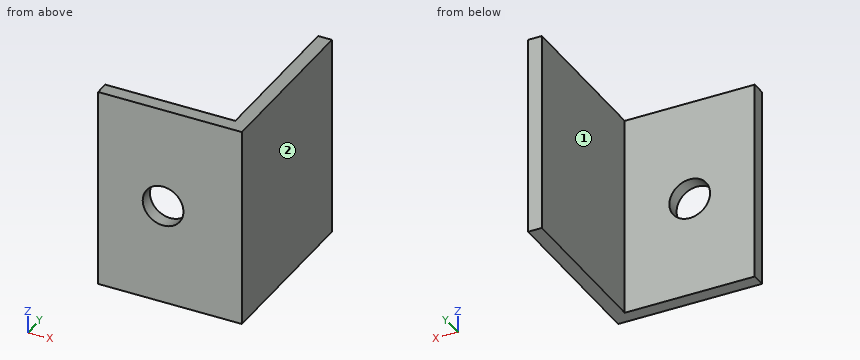
from build123d import *

# Parameters (mm, degrees)
BOSS_EXTRUDE1_DEPTH       = 11.1125
F_8_CLEARANCE_HOLE1_D     = 4.4958
F_8_CLEARANCE_HOLE1_DEPTH = 31.75
F_8_CLEARANCE_HOLE1_TIP   = 1.350674586


with BuildPart() as part:
    # Sketch1 → Boss-Extrude1 (new, symmetric)
    with BuildSketch(Plane.XY):
        Polygon((-14.351, 0), (0, 0), (0, 17.526), (1.524, 17.526), (1.524, -1.524), (-14.351, -1.524), align=None)
    extrude(amount=BOSS_EXTRUDE1_DEPTH, both=True)

    # #8 Clearance Hole1
    with Locations(Plane(origin=(0, 0, 0), x_dir=(1, 0, 0), z_dir=(0, 1, 0))):
        with Locations((-7.1755, 0)):
            Hole(F_8_CLEARANCE_HOLE1_D / 2, depth=F_8_CLEARANCE_HOLE1_DEPTH)
            with Locations((0, 0, -(F_8_CLEARANCE_HOLE1_DEPTH + F_8_CLEARANCE_HOLE1_TIP / 2))):  # 118° drill point
                Cone(0, F_8_CLEARANCE_HOLE1_D / 2, F_8_CLEARANCE_HOLE1_TIP, mode=Mode.SUBTRACT)


solid = part.part
Work out the finished part from the listing and answer in its coordinate system (mm). Face numbers are marked on the shaded views. A direction names the side the tool comes from. Coordinates: 2 decimals unless noted, no trailing zeros. Loops run counter-clockwise (first coordinate to the right, second up) from the corner with the lowest first, then second, coordinate; pieces in that order, holes last. Notation, with made-up numbers: M 52,-0.75 L 86,-0.75 A19 cw 86,7.25 Z; hole C 29.5,67 d3. An arc over 180 degrees is marked long. Answer in a Markdown table with one row per item. Add a question column.
1. A tool of negligible diameter and unlimited length cuts with its end or side. For the marked faces 1 and 2, from which of +Z, -Z, +X, -X, +Y, -Y can it reach the whole face along a straight path? Write none if from no direction.
2. Find section C-C, the plane z = -6.5. Write down the section's boundary in (x, y).
3. Consider L1, parallel to Y at x = -7, z = 3; L2, parallel to X at y = 15, z = 7; L3, parallel to Z at x = -6, y = -0.5. Determine where each line is inside the solid, lowest interval first.
4. Flat-ended cylindrical pins translate along their axes: P1, Ø6, axis at x = -9, z = -4.5, coming from the +Y side; P2, Ø1.5, axis at x = -9.5, y = 1, coming from the -Z side; P3, Ø5.5, axis at y = 5, z = 5, coming from the -X side. Find the tip coordinate at first contact, or state that the pin passes through.
5. Find section D-D, the plane y = 5.75. Write down the section's boundary in (x, z).
6. Find section B-B, the plane x = -6.5. Write down the section's boundary in (y, z).
7. Find section A-A, the plane z = 0. Write down the section's boundary in (x, y).
Reported:
| question | item | result |
|---|---|---|
| 1 | face 1 | +Z, -Z, -X, +Y |
| 1 | face 2 | +Z, -Z, +X, +Y, -Y |
| 2 | outline | M -14.35,-1.52 L 1.52,-1.52 L 1.52,17.53 L 0,17.53 L 0,0 L -14.35,0 Z |
| 3 | L1 | y = -1.52 to 0 |
| 3 | L2 | x = 0 to 1.52 |
| 3 | L3 | z = -11.11 to -1.92, 1.92 to 11.11 |
| 4 | P1 | stops at y = 0 |
| 4 | P2 | passes through |
| 4 | P3 | stops at x = 0 |
| 5 | outline | M 0,-11.11 L 1.52,-11.11 L 1.52,11.11 L 0,11.11 Z |
| 6 | outline | M -1.52,-11.11 L 0,-11.11 L 0,-2.14 L -1.52,-2.14 Z; M -1.52,2.14 L 0,2.14 L 0,11.11 L -1.52,11.11 Z |
| 7 | outline | M -14.35,-1.52 L -9.42,-1.52 L -9.42,0 L -14.35,0 Z; M -4.93,-1.52 L 1.52,-1.52 L 1.52,17.53 L 0,17.53 L 0,0 L -4.93,0 Z |
